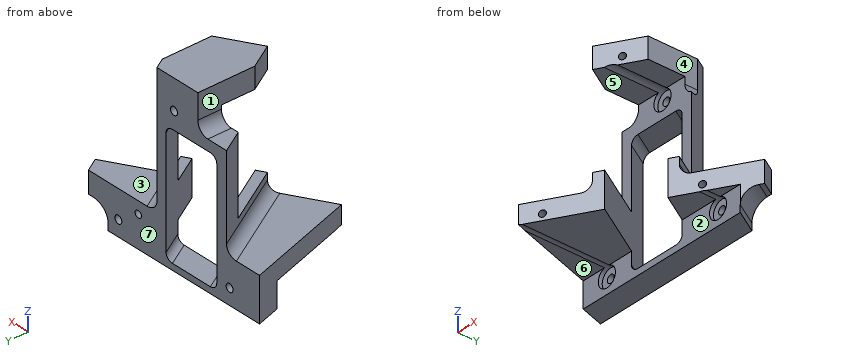
from build123d import *

# Parameters (mm, degrees)
PAD_DEPTH         = 88
SKETCH001_R       = 2
POCKET_DEPTH      = 0.001
POCKET_DEPTH_BACK = 57.033261
SKETCH002_R       = 5
POCKET001_DEPTH   = 47.033261
SKETCH003_R       = 1.65
POCKET002_DEPTH   = 28
POCKET003_DEPTH   = 58.134580172
POCKET004_DEPTH   = 45.033261


with BuildPart() as part:
    # Sketch → Pad (new body)
    with BuildSketch(Plane.XY):
        Polygon((0, 0), (-50, 0), (-32.5156133784, -57.032261), (54.086927, -7.032261), (50, 0), align=None)
    extrude(amount=PAD_DEPTH)

    # Sketch001 → Pocket (cut, two sides)
    with BuildSketch(Plane.XZ) as pocket_sk:
        with Locations((-32.5, 8)):
            Circle(SKETCH001_R)
        with Locations((32.5, 8)):
            Circle(SKETCH001_R)
        with Locations((0, 73)):
            Circle(SKETCH001_R)
        with BuildLine():
            ThreePointArc((-31.448877, 94.382629), (-35.5661724156, 92.6771893986), (-37.2716120171, 88.5598939829))
            Line((-37.2716120171, 75.5089300171), (-37.2716120171, 88.5598939829))
            ThreePointArc((-37.2716120171, 75.5089300171), (-35.5661724156, 71.3916346014), (-31.448877, 69.686195))
            Line((-19.8034130171, 69.686195), (-31.448877, 69.686195))
            ThreePointArc((-19.8034130171, 69.686195), (-15.6861176014, 71.3916346014), (-13.980678, 75.5089300171))
            Line((-13.980678, 88.5598939829), (-13.980678, 75.5089300171))
            ThreePointArc((-13.980678, 88.5598939829), (-15.6861176014, 92.6771893986), (-19.8034130171, 94.382629))
            Line((-31.448877, 94.382629), (-19.8034130171, 94.382629))
        make_face()
        with BuildLine():
            ThreePointArc((18.49613, 98.398308), (14.6982792772, 96.8251867228), (13.125158, 93.027336))
            Line((13.125158, 73.852471), (13.125158, 93.027336))
            ThreePointArc((13.125158, 73.852471), (14.6982792772, 70.0546202772), (18.49613, 68.481499))
            Line((29.238075, 68.481499), (18.49613, 68.481499))
            ThreePointArc((29.238075, 68.481499), (33.0359257228, 70.0546202772), (34.609047, 73.852471))
            Line((34.609047, 93.027336), (34.609047, 73.852471))
            ThreePointArc((34.609047, 93.027336), (33.0359257228, 96.8251867228), (29.238075, 98.398308))
            Line((18.49613, 98.398308), (29.238075, 98.398308))
        make_face()
    extrude(amount=-POCKET_DEPTH, mode=Mode.SUBTRACT)
    extrude(pocket_sk.sketch, amount=POCKET_DEPTH_BACK, mode=Mode.SUBTRACT)

    # Sketch002 → Pocket001 (cut, through all)
    with BuildSketch(Plane.XZ.offset(10)):
        with Locations((-32.5, 8)):
            Circle(SKETCH002_R)
        with Locations((32.5, 8)):
            Circle(SKETCH002_R)
        with Locations((0, 73)):
            Circle(SKETCH002_R)
    extrude(amount=POCKET001_DEPTH, mode=Mode.SUBTRACT)

    # Sketch003 (on Face2 of Pocket001) → Pocket002 (cut)
    with BuildSketch(Plane(origin=(16.566790086, -28.6945221473, 0), x_dir=(0.8660254038, 0.5, 0), z_dir=(0.5, -0.8660254038, 0))):
        with Locations((18.0690987246, 16)):
            Circle(SKETCH003_R)
        with Locations((-46.9309012754, 16)):
            Circle(SKETCH003_R)
        with Locations((-14.4309012754, 81)):
            Circle(SKETCH003_R)
    extrude(amount=-POCKET002_DEPTH, mode=Mode.SUBTRACT)

    # Sketch004 (on Face2 of Pocket002) → Pocket003 (cut, through all)
    with BuildSketch(Plane(origin=(16.566790086, -28.6945221473, 0), x_dir=(0.8660254038, 0.5, 0), z_dir=(0.5, -0.8660254038, 0))):
        with BuildLine():
            ThreePointArc((13.6215579788, 99.375281956), (10.0860240728, 97.9108158619), (8.6215579788, 94.375281956))
            Line((8.6215579788, 27.1252926568), (8.6215579788, 94.375281956))
            ThreePointArc((8.6215579788, 27.1252926568), (10.0860240728, 23.5897587509), (13.6215579788, 22.1252926568))
            Line((44.7393771197, 22.1252926568), (13.6215579788, 22.1252926568))
            ThreePointArc((44.7393771197, 22.1252926568), (48.2749110256, 23.5897587509), (49.7393771197, 27.1252926568))
            Line((49.7393771197, 94.375281956), (49.7393771197, 27.1252926568))
            ThreePointArc((49.7393771197, 94.375281956), (48.2749110256, 97.9108158619), (44.7393771197, 99.375281956))
            Line((13.6215579788, 99.375281956), (44.7393771197, 99.375281956))
        make_face()
        with BuildLine():
            ThreePointArc((-82.3406850147, 105.6353147348), (-85.8762189206, 104.1708486408), (-87.3406850147, 100.6353147348))
            Line((-87.3406850147, 27.1252928143), (-87.3406850147, 100.6353147348))
            ThreePointArc((-87.3406850147, 27.1252928143), (-85.8762189206, 23.5897589083), (-82.3406850147, 22.1252928143))
            Line((-31.5974694977, 22.1252928143), (-82.3406850147, 22.1252928143))
            ThreePointArc((-31.5974694977, 22.1252928143), (-28.0619355917, 23.5897589083), (-26.5974694977, 27.1252928143))
            Line((-26.5974694977, 100.6353147348), (-26.5974694977, 27.1252928143))
            ThreePointArc((-26.5974694977, 100.6353147348), (-28.0619355917, 104.1708486408), (-31.5974694977, 105.6353147348))
            Line((-82.3406850147, 105.6353147348), (-31.5974694977, 105.6353147348))
        make_face()
        with BuildLine():
            ThreePointArc((-18.4163422765, 64.182594), (-20.6977909978, 63.2375869978), (-21.642798, 60.9561382765))
            Line((-21.642798, 6.4200485882), (-21.642798, 60.9561382765))
            ThreePointArc((-21.642798, 6.4200485882), (-20.6977909978, 4.1385998669), (-18.4163422765, 3.1935928646))
            Line((0.7763344118, 3.1935928646), (-18.4163422765, 3.1935928646))
            ThreePointArc((0.7763344118, 3.1935928646), (3.0577831331, 4.1385998669), (4.0027901354, 6.4200485882))
            Line((4.0027901354, 60.9561382765), (4.0027901354, 6.4200485882))
            ThreePointArc((4.0027901354, 60.9561382765), (3.0577831331, 63.2375869978), (0.7763344118, 64.182594))
            Line((-18.4163422765, 64.182594), (0.7763344118, 64.182594))
        make_face()
        with BuildLine():
            ThreePointArc((33.371799, -13.9859969869), (35.6183005855, -19.4095315824), (41.041835181, -21.6560331679))
            Line((57.2190858452, -21.6560331679), (41.041835181, -21.6560331679))
            ThreePointArc((57.2190858452, -21.6560331679), (62.6426204407, -19.4095315824), (64.8891220262, -13.9859969869))
            Line((64.8891220262, 3.485097), (64.8891220262, -13.9859969869))
            ThreePointArc((64.8891220262, 3.485097), (62.6426204407, 8.9086315955), (57.2190858452, 11.155133181))
            Line((41.041835181, 11.155133181), (57.2190858452, 11.155133181))
            ThreePointArc((41.041835181, 11.155133181), (35.6183005855, 8.9086315955), (33.371799, 3.485097))
            Line((33.371799, -13.9859969869), (33.371799, 3.485097))
        make_face()
    extrude(amount=-POCKET003_DEPTH, mode=Mode.SUBTRACT)

    # Sketch005 → Pocket004 (cut, through all)
    with BuildSketch(Plane.XZ.offset(12)):
        with BuildLine():
            ThreePointArc((-72.562921396, 12.818138604), (-85.0985797487, 7.625698901), (-90.2910194516, -4.9099594516))
            Line((-90.2910194516, -39.9313305758), (-90.2910194516, -4.9099594516))
            ThreePointArc((-90.2910194516, -39.9313305758), (-85.0985797487, -52.4669889284), (-72.562921396, -57.6594286314))
            Line((82.146623396, -57.6594286314), (-72.562921396, -57.6594286314))
            ThreePointArc((82.146623396, -57.6594286314), (94.6822817487, -52.4669889284), (99.8747214516, -39.9313305758))
            Line((99.8747214516, -4.9099594516), (99.8747214516, -39.9313305758))
            ThreePointArc((99.8747214516, -4.9099594516), (94.6822817487, 7.625698901), (82.146623396, 12.818138604))
            Line((-72.562921396, 12.818138604), (82.146623396, 12.818138604))
        make_face()
        with BuildLine():
            ThreePointArc((-53.674213, 77.4039000645), (-62.7743204587, 73.6345121361), (-66.5437083871, 64.5344046774))
            Line((-66.5437083871, 43.4490521935), (-66.5437083871, 64.5344046774))
            ThreePointArc((-66.5437083871, 43.4490521935), (-62.7743204587, 34.3489447349), (-53.674213, 30.5795568065))
            Line((56.105189, 30.5795568065), (-53.674213, 30.5795568065))
            ThreePointArc((56.105189, 30.5795568065), (65.2052964587, 34.3489447349), (68.9746843871, 43.4490521935))
            Line((68.9746843871, 64.5344046774), (68.9746843871, 43.4490521935))
            ThreePointArc((68.9746843871, 64.5344046774), (65.2052964587, 73.6345121361), (56.105189, 77.4039000645))
            Line((-53.674213, 77.4039000645), (56.105189, 77.4039000645))
        make_face()
    extrude(amount=POCKET004_DEPTH, mode=Mode.SUBTRACT)


solid = part.part
Work out the finished part from the listing and answer in its coordinate system (mm). Face numbers are marked on the shaded views. A direction names the side the tool comes from. Coordinates: 2 decimals unless noted, no trailing zeros. Loops run counter-clockwise (first coordinate to the right, second up) from the corner with the lowest first, then second, coordinate; pieces in that order, holes last. Notation, with made-up numbers: (-28.5, 61) -> (22.5, 61) arc R23 ccw to (22.5, 69) -> close; hole circle Ø8 at (9, 27). An arc over 180 degrees is marked (long way). Write each question's results on one line, items separated by ' | '. Start each with the question number.
1) Find section A-A on z = 62.5. Determine the outline of the cut face in (x, y), then the cut area to 3 significant figures.
2) Flat-ended cylindrical pins translate along their axes: P1, Ø16, axis at x = 0, z = 73, coming from the -Y side; P2, Ø8, axis at y = -12, z = 50, coming from the -X side; P3, Ø11.5, axis at y = -24, z = 81, coming from the +X side; P4, Ø10, axis at x = 18, y = -19.5, coming from the +Z side. Find the tip coordinate at first contact, or state that the pin passes through.
3) Consider line 1 along Z through (x, y) = (0, -3.25); line 2 along Y through (x, z) = (3.5, 68); line 3 along Z through (x, y) = (32.5, -13.25). Determine where each line is inside the solid, lowest interval first.
4) Find section B-B on z = 8. Determine the outline of the cut face in (x, y), then the cut area to 3 significant figures.
5) For the marked faces 1, 2, 3 and 4, determine the directions among +Z, -Z, +X, -X, +Y, -Y from which every point of the face is accessible in a straight line to the end or side of a thin tool.
6) Find section C-C on y = -32. Count the separate pieces of the cut face and the enclosed holes in it, then the cut area to 3 significant figures.
7) The mould has two halves that part along Z. Classify the marked faces 5, 6 and 7: pulls with the +Z half, pulls with the -Z half, needs draft (parallel to the pull), parting line crosses it, or undercut.
Response values:
1) outline: (-30.71, 0) -> (-23.78, -12) -> (-17.61, -12) -> (-24.54, 0) -> close; (4.17, 0) -> (11.1, -12) -> (16.88, -12) -> (9.96, 0) -> close | area: 144 mm^2
2) P1: stops at y = -41.99 | P2: stops at x = -26.09 | P3: stops at x = 13.13 | P4: stops at z = 88
3) line 1: z = 0 to 3.19, 64.18 to 71, 75 to 88 | line 2: y = -12 to 0 | line 3: z = 13 to 22.13
4) outline: (-50, 0) -> (-46.32, -12) -> (-37.5, -12) -> (-37.5, -10) -> (-34.5, -10) -> (-34.5, 0) -> close; (-30.5, -10) -> (-27.5, -10) -> (-27.5, -12) -> (-18.06, -12) -> (-24.99, 0) -> (-30.5, 0) -> close; (4.62, 0) -> (11.55, -12) -> (27.5, -12) -> (27.5, -10) -> (30.5, -10) -> (30.5, 0) -> close; (34.5, -10) -> (37.5, -10) -> (37.5, -12) -> (45.48, -12) -> (46.74, -11.27) -> (40.23, 0) -> (34.5, 0) -> close | area: 626 mm^2
5) face 1: +Z, -X, +Y, -Y | face 2: -Z, +X, -X, -Y | face 3: +Z, +X, +Y | face 4: +Z, +X, +Y, -Y
6) separate pieces: 2 | enclosed holes: 2 | area: 591 mm^2
7) face 5: undercut | face 6: pulls with the -Z half | face 7: needs draft
